Check sheet for the modelled part. Datum: model origin and axes. Units: mm. A direction names the side the tool comes from. Round coordinates to 2 decimals unless told otherwise and drop trailing zeros. Order: outer loops, then holes, each group sorted by start corner. A loop starts at its lowest first (then second) coordinate and runs counter-clockwise, first axis right, second up. Notation, with made-up numbers: (-37.5, 79) -> (-11.5, 79) arc R12 ccw to (-11.5, 93) -> close; hole circle Ø6 at (54, -7.75). An arc over 180 degrees is marked (long way). Answer in a Markdown table with one row per item.
```python
from build123d import *

# Parameters (mm, degrees)
ESQUISSE1_R        = 2.5
BOSS_EXTRU_1_DEPTH = 5
CONG_1_R           = 10


with BuildPart() as part:
    # Esquisse1 → Boss.-Extru.1 (new body)
    with BuildSketch(Plane.XY):
        Polygon((-31.5, -3), (-32.6, -3), (-32.6, -5.3), (-31.5, -5.3), (-31.5, -10), (-28.5, -10), (-28.5, -5.3), (-27.4, -5.3), (-27.4, -3), (-28.5, -3), (-28.5, 0), (-25, 0), (-25, 5), (-20, 5), (-20, 0), (-20, -20), (20, -20), (20, 0), (20, 5), (25, 5), (25, 0), (28.5, 0), (28.5, -3), (27.4, -3), (27.4, -5.3), (28.5, -5.3), (28.5, -10), (31.5, -10), (31.5, -5.3), (32.6, -5.3), (32.6, -3), (31.5, -3), (31.5, 0), (35, 0), (35, 5), (40, 5), (40, 0), (40, -40), (-40, -40), (-40, 0), (-40, 5), (-35, 5), (-35, 0), (-31.5, 0), align=None)
        with Locations((30, -35)):
            Circle(ESQUISSE1_R, mode=Mode.SUBTRACT)
        with Locations((-30, -35)):
            Circle(ESQUISSE1_R, mode=Mode.SUBTRACT)
    extrude(amount=BOSS_EXTRU_1_DEPTH)

    # Congé1
    cong_1_edges = [part.edges().sort_by_distance(p)[0] for p in [
        (-20, -20, 2.5),
        (20, -20, 2.5),
        (40, -40, 2.5),
        (-40, -40, 2.5),
    ]]
    fillet(cong_1_edges, radius=CONG_1_R)


solid = part.part
```
(1) Section check C-C on z = 2.45. Give the number of separate pieces and of enclosed holes in the cut face, plus the area to 3 significant figures.
Solutions:
| item | result |
|---|---|
| separate pieces | 1 |
| enclosed holes | 2 |
| area | 2,390 mm^2 |
(2) Draft check along X on faces 4 (the flat face through (-28.5, -2, 2)), 5 (the cylindrical face through (36.99, -37.15, 2.54)), 6 (the flat face through (22, 5, 2)). Enter one of: pulls with the +X half, pulls with the -X half, needs draft (parallel to the pull), parting line crosses it, or undercut.
Solutions:
| item | result |
|---|---|
| face 4 | undercut |
| face 5 | pulls with the +X half |
| face 6 | needs draft |
(3) Section check D-D on y = -14. Record the boundary of the cut face in (x, z).
Solutions:
| item | result |
|---|---|
| outline | (-40, 0) -> (-19.17, 0) -> (-19.17, 5) -> (-40, 5) -> close; (19.17, 0) -> (40, 0) -> (40, 5) -> (19.17, 5) -> close |
(4) Section check B-B on y = -35. Record the boundary of the cut face in (x, z).
Solutions:
| item | result |
|---|---|
| outline | (-38.66, 0) -> (-32.5, 0) -> (-32.5, 5) -> (-38.66, 5) -> close; (-27.5, 0) -> (27.5, 0) -> (27.5, 5) -> (-27.5, 5) -> close; (32.5, 0) -> (38.66, 0) -> (38.66, 5) -> (32.5, 5) -> close |
(5) Depth check by flat-ended pin: pin 1 Ø1.5 at (x, z) = (30.5, 1.5) entering from +Y; pin 2 Ø8 at (x, y) = (30, -35) entering from +Z; pin 3 Ø0.6 at (x, z) = (28, 2.5) entering from +Y. Enter the tip coordinate at first touch or a pass-through.
Solutions:
| item | result |
|---|---|
| pin 1 | y = -10 |
| pin 2 | z = 5 |
| pin 3 | y = 0 |
(6) Scan lines: probe 1 along X at (y, z) = (-4, 3.1); probe 2 along X at (y, z) = (2, 0.35); probe 3 along X at (y, z) = (-10.5, 3.2). Record each from-to range of solid material in increasing order. Write a range as from..to.
Solutions:
| item | result |
|---|---|
| probe 1 | -40..-32.6, -27.4..-20, 20..27.4, 32.6..40 |
| probe 2 | -40..-35, -25..-20, 20..25, 35..40 |
| probe 3 | -40..-19.99, 19.99..40 |
(7) Section check A-A on y = -6.5. Record the boundary of the cut face in (x, z), plus the area to 3 significant figures.
Solutions:
| item | result |
|---|---|
| outline | (-40, 0) -> (-31.5, 0) -> (-31.5, 5) -> (-40, 5) -> close; (-28.5, 0) -> (-20, 0) -> (-20, 5) -> (-28.5, 5) -> close; (20, 0) -> (28.5, 0) -> (28.5, 5) -> (20, 5) -> close; (31.5, 0) -> (40, 0) -> (40, 5) -> (31.5, 5) -> close |
| area | 170 mm^2 |
(8) Tool access check on faces 1 (the flat face through (20, -2, 2)), 2 (the flat face through (37, 5, 2)), 3 (the flat face through (27.4, -4, 2)). Record the directions out of +Z, -Z, +X, -X, +Y, -Y that give a thin tool (end or side, any length) a straight path to the whole face; none if there is none.
Solutions:
| item | result |
|---|---|
| face 1 | +Z, -Z, +Y |
| face 2 | +Z, -Z, +X, -X, +Y |
| face 3 | +Z, -Z |
